Verification items for the finished model (mm, model axes). A direction names the side the tool comes from. Round coordinates to 2 decimals unless told otherwise and drop trailing zeros. Order: outer loops, then holes, each group sorted by start corner. A loop starts at its lowest first (then second) coordinate and runs counter-clockwise, first axis right, second up. Notation, with made-up numbers: (61.25, 74.25) -> (74.25, 74.25) arc R18 ccw to (74.25, 90.25) -> close; hole circle Ø1 at (47.25, -30.75). An arc over 180 degrees is marked (long way). Put each result on its own line as item: value.
```python
from build123d import *

# Parameters (mm, degrees)
ESQUISSE1_W        = 90
ESQUISSE1_H        = 10
BOSS_EXTRU_1_DEPTH = 10


with BuildPart() as part:
    # Esquisse1 → Boss.-Extru.1 (new body)
    with BuildSketch(Plane.XY):
        Polygon((0, 170), (598, 170), (598, 0), (598, -50), (558, -50), (498, 0), (100, 0), (40, -50), (0, -50), (0, 0), align=None)
        with Locations((224, 125)):
            Rectangle(ESQUISSE1_W, ESQUISSE1_H, mode=Mode.SUBTRACT)
        with Locations((374, 125)):
            Rectangle(ESQUISSE1_W, ESQUISSE1_H, mode=Mode.SUBTRACT)
        with Locations((74, 125)):
            Rectangle(ESQUISSE1_W, ESQUISSE1_H, mode=Mode.SUBTRACT)
        with Locations((524, 125)):
            Rectangle(ESQUISSE1_W, ESQUISSE1_H, mode=Mode.SUBTRACT)
    extrude(amount=BOSS_EXTRU_1_DEPTH)


solid = part.part
```
Item 1: Sectioned sample at C-C, the plane z = 1.5. Record the boundary of the cut face in (x, y), then the cut area to 3 significant figures.
Geometry check:
outline: (0, -50) -> (40, -50) -> (100, 0) -> (498, 0) -> (558, -50) -> (598, -50) -> (598, 170) -> (0, 170) -> close; hole (29, 120) -> (119, 120) -> (119, 130) -> (29, 130) -> close; hole (179, 120) -> (269, 120) -> (269, 130) -> (179, 130) -> close; hole (329, 120) -> (419, 120) -> (419, 130) -> (329, 130) -> close; hole (479, 120) -> (569, 120) -> (569, 130) -> (479, 130) -> close
area: 105,000 mm2
Item 2: Sectioned sample at A-A, the plane x = 490.5. Record the boundary of the cut face in (y, z).
Geometry check:
outline: (0, 0) -> (120, 0) -> (120, 10) -> (0, 10) -> close; (130, 0) -> (170, 0) -> (170, 10) -> (130, 10) -> close
Item 3: Tool access check on faces 4 (the face through (523, 120, 5)), 5 (the face through (528, -25, 5)), 6 (the face through (20, -50, 5)). Record the directions out of +Z, -Z, +X, -X, +Y, -Y that give a thin tool (end or side, any length) a straight path to the whole face; none if there is none.
Geometry check:
face 4: +Z, -Z
face 5: +Z, -Z, -Y
face 6: +Z, -Z, +X, -X, -Y
Item 4: Depth check by flat-ended pin: pin 1 Ø6 at (x, y) = (533.5, 37) entering from -Z; pin 2 Ø5 at (x, z) = (239, 4) entering from -Y; pin 3 Ø5 at (x, z) = (527.5, 6.5) entering from -Y; pin 4 Ø3 at (x, z) = (517.5, 6) entering from -Y. Enter the tip coordinate at first touch or a pass-through.
Geometry check:
pin 1: z = 0
pin 2: y = 0
pin 3: y = -26.67
pin 4: y = -17.5
Item 5: Material ranges on line 1 along Y through (x, z) = (104.5, 6); line 2 along Y through (x, z) = (56.5, 6.5), recorded low to high.
Geometry check:
line 1: 0 to 120, 130 to 170
line 2: -36.25 to 120, 130 to 170
Item 6: Sectioned sample at B-B, the plane y = -19.5. Record the boundary of the cut face in (x, z).
Geometry check:
outline: (0, 0) -> (76.6, 0) -> (76.6, 10) -> (0, 10) -> close; (521.4, 0) -> (598, 0) -> (598, 10) -> (521.4, 10) -> close
Item 7: Release check for a two-part mould opening along Y. For faces 1 (the face through (578, -50, 5)), 2 (the face through (303, 86, 10)), 3 (the face through (179, 125, 5)) record: pulls with the +Y half, pulls with the -Y half, needs draft (parallel to the pull), parting line crosses it, or undercut.
Geometry check:
face 1: pulls with the -Y half
face 2: needs draft
face 3: undercut
